```python
from build123d import *

# Parameters (mm, degrees)
BOSS_EXTRUDE1_DEPTH = 34.2
SKETCH2_R           = 8
CUT_EXTRUDE1_DEPTH  = 10
SKETCH3_W           = 21.2
SKETCH3_H           = 36.6
BOSS_EXTRUDE2_DEPTH = 2
SKETCH5_R           = 1.65
CUT_EXTRUDE4_DEPTH  = 78.321407126


with BuildPart() as part:
    # Sketch1 → Boss-Extrude1 (new body)
    with BuildSketch(Plane.XY):
        Polygon((0, 38.5), (19.5, 53.6), (42, 53.6), (42, 0), (0, 0), align=None)
    extrude(amount=BOSS_EXTRUDE1_DEPTH)

    # Sketch2 → Cut-Extrude1 (cut)
    with BuildSketch(Plane.XZ):
        with Locations(Location((26, 23.7, 0), (0, 0, 270))):
            Circle(SKETCH2_R)
    extrude(amount=-CUT_EXTRUDE1_DEPTH, mode=Mode.SUBTRACT)

    # Sketch3 → Boss-Extrude2 (add)
    with BuildSketch(Plane(origin=(42, 0, 0), x_dir=(0, 0, -1), z_dir=(1, 0, 0))):
        with Locations((-19.1, 35.3)):
            Rectangle(SKETCH3_W, SKETCH3_H)
    extrude(amount=BOSS_EXTRUDE2_DEPTH)

    # Sketch5 → Cut-Extrude4 (cut, through all)
    with BuildSketch(Plane(origin=(0, 0, 0), x_dir=(-1, 0, 0), z_dir=(0, 0, -1))):
        with Locations((-36, 5)):
            Circle(SKETCH5_R)
        with Locations((-5, 5)):
            Circle(SKETCH5_R)
        with Locations((-5, 36)):
            Circle(SKETCH5_R)
    extrude(amount=-CUT_EXTRUDE4_DEPTH, mode=Mode.SUBTRACT)


solid = part.part
```
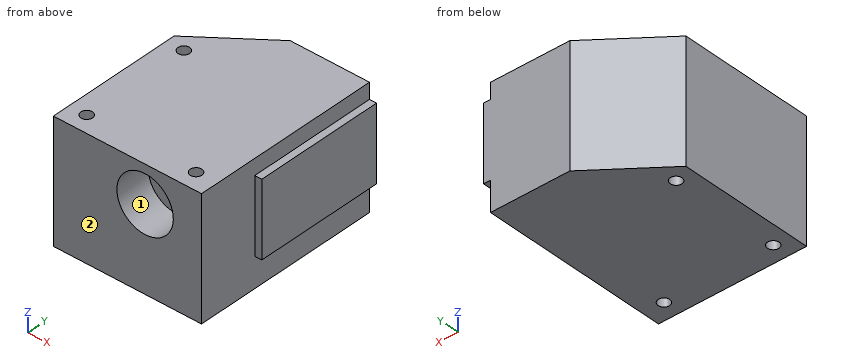
Build history of the part. All positions in model axes, mm. Face numbers are marked on the shaded views. A direction names the side the tool comes from. Coordinates: 2 decimals unless noted, no trailing zeros. Order: outer loops, then holes, each group sorted by start corner. A loop starts at its lowest first (then second) coordinate and runs counter-clockwise, first axis right, second up. Notation, with made-up numbers: (-24, 89) -> (28, 89) arc R18 ccw to (28, 107) -> close; hole circle Ø1 at (78.25, 71.25). An arc over 180 degrees is marked (long way). Answer in a Markdown table with one row per item. Add a question column.
Q1. Band-saw the part on A-A, the plane x = 36. List the corners of the cut face in (y, z).
Q2. Band-saw the part on C-C, the plane z = 23.7. List the corners of the cut face in (x, y), then the cut area to 3 significant figures.
Q3. Wall check: line 1 along Y through (x, z) = (4, 19); line 2 along Y through (x, z) = (36, 16); line 3 along X through (y, z) = (6, 23.7). Give the ranges that are in metal, low to high. Write a range as [from, to].
Q4. Which spindle directions (+Z, -Z, +X, -X, +Y, -Y) get a long thin tool onto all of the face, cutting with end or side? Do the marked faces 1 and 2. Say none if no direction does.
Q5. Drop flat-ended pins along their axis: pin 1 (12 mm diameter, centred on x = 9.5, z = 21.5, fed in from +Y); pin 2 (3 mm diameter, centred on y = 6, z = 13.5, fed in from +X); pin 3 (0.6 mm diameter, centred on x = 43, z = 19, fed in from -Y). Give the stop position or say it passes through.
Q6. Band-saw the part on D-D, the plane x = 4. List the corners of the cut face in (y, z).
Q7. Band-saw the part on B-B, the plane y = 36. List the corners of the cut face in (x, z), then the cut area to 3 significant figures.
Answers follow:
| question | item | result |
|---|---|---|
| 1 | outline | (0, 0) -> (3.35, 0) -> (3.35, 34.2) -> (0, 34.2) -> close; (6.65, 0) -> (53.6, 0) -> (53.6, 34.2) -> (6.65, 34.2) -> close |
| 2 | outline | (0, 0) -> (18, 0) -> (18, 10) -> (34, 10) -> (34, 0) -> (42, 0) -> (42, 17) -> (44, 17) -> (44, 53.6) -> (19.5, 53.6) -> (0, 38.5) -> close; hole circle Ø3.3 at (5, 5); hole circle Ø3.3 at (5, 36); hole circle Ø3.3 at (36, 5) |
| 2 | area | 1,990 mm^2 |
| 3 | line 1 | [0, 3.69], [6.31, 34.69], [37.31, 41.6] |
| 3 | line 2 | [0, 3.35], [6.65, 53.6] |
| 3 | line 3 | [0, 3.69], [6.31, 18], [34, 34.69], [37.31, 42] |
| 4 | face 1 | -Y |
| 4 | face 2 | +Z, -Z, +X, -X, -Y |
| 5 | pin 1 | y = 50.5 |
| 5 | pin 2 | x = 42 |
| 5 | pin 3 | y = 17 |
| 6 | outline | (0, 0) -> (3.69, 0) -> (3.69, 34.2) -> (0, 34.2) -> close; (6.31, 0) -> (34.69, 0) -> (34.69, 34.2) -> (6.31, 34.2) -> close; (37.31, 0) -> (41.6, 0) -> (41.6, 34.2) -> (37.31, 34.2) -> close |
| 7 | outline | (0, 0) -> (3.35, 0) -> (3.35, 34.2) -> (0, 34.2) -> close; (6.65, 0) -> (42, 0) -> (42, 8.5) -> (44, 8.5) -> (44, 29.7) -> (42, 29.7) -> (42, 34.2) -> (6.65, 34.2) -> close |
| 7 | area | 1,370 mm^2 |
